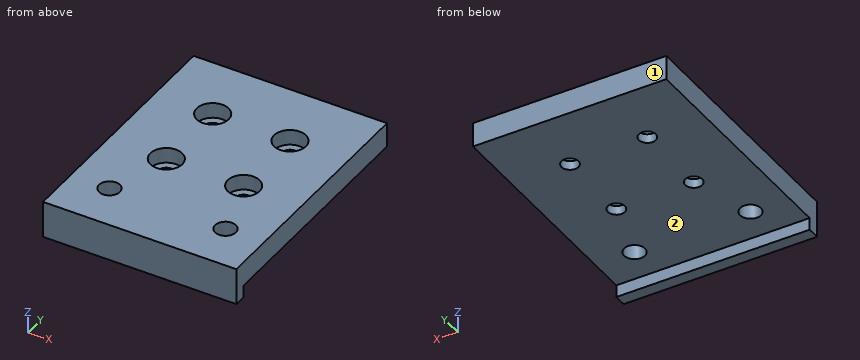
```python
from build123d import *

# Parameters (mm, degrees)
F0_W           = 50
F0_H           = 65
F1_DEPTH       = 9.525
F2_W           = 50
F2_H           = 61.825
F3_DEPTH       = 3.175
F5_D           = 4.4
F5_CBORE_D     = 8.25
F5_CBORE_DEPTH = 4
F7_D           = 5.4


# Not quite as in the source:
# - a length typed as a fraction of an inch, garbled in the dataset ("3 / 203.2 mm" for 3/8 in), is restored


with BuildPart() as f1:
    # F0 (on Top) → F1 (new body)
    with BuildSketch(Plane.XY):
        Rectangle(F0_W, F0_H)
    extrude(amount=F1_DEPTH)

    # F2 (on face) → F3 (cut)
    with BuildSketch(Plane(origin=(0, 0, 0), x_dir=(1, 0, 0), z_dir=(0, 0, -1))):
        with Locations((0, -1.5875)):
            Rectangle(F2_W, F2_H)
    extrude(amount=-F3_DEPTH, mode=Mode.SUBTRACT)

    # F5 (through all)
    with Locations(Plane.XY.offset(9.525)):
        with Locations((-10, 15.675), (10, 15.675), (10, -4.325), (-10, -4.325)):
            CounterBoreHole(F5_D / 2, F5_CBORE_D / 2, F5_CBORE_DEPTH)

    # F7 (through all)
    with Locations(Plane.XY.offset(9.525)):
        with Locations((-15, -20.5), (15, -20.5)):
            Hole(F7_D / 2)


solid = f1.part
```
Verification items for the finished model (mm, model axes). Face numbers are marked on the shaded views. A direction names the side the tool comes from. Coordinates: 2 decimals unless noted, no trailing zeros. Loops run counter-clockwise (first coordinate to the right, second up) from the corner with the lowest first, then second, coordinate; pieces in that order, holes last. Notation, with made-up numbers: (-24.75, -35.75) - (-11.75, -35.75) arc R22 cw to (-11.75, -29.75) - close; hole circle Ø7 at (-8.5, 29.25). An arc over 180 degrees is marked (long way). Answer as a JSON object with one key per item and string values.
(1) Access from +Z, -Z, +X, -X, +Y, -Y to the whole of each face (thin tool, end or side, straight path). Record for the marked faces 1 and 2.
Response:
{"face 1": "+Z, -Z, +X, -X, +Y", "face 2": "-Z, +X, -X, +Y"}
(2) Cross-section at D-D, the plane z = 4.5. Record the boundary of the cut face in (x, y) (3 decimals), then the cut area to 3 significant figures.
Response:
{"outline": "(-25, -32.5) - (25, -32.5) - (25, 32.5) - (-25, 32.5) - close; hole circle Ø5.4 at (-15, -20.5); hole circle Ø4.4 at (-10, -4.325); hole circle Ø4.4 at (-10, 15.675); hole circle Ø4.4 at (10, -4.325); hole circle Ø4.4 at (10, 15.675); hole circle Ø5.4 at (15, -20.5)", "area": "3,140 mm²"}
(3) Cross-section at A-A, the plane y = -20.5. Record the boundary of the cut face in (x, z) (3 decimals).
Response:
{"outline": "(-25, 3.175) - (-17.7, 3.175) - (-17.7, 9.525) - (-25, 9.525) - close; (-12.3, 3.175) - (12.3, 3.175) - (12.3, 9.525) - (-12.3, 9.525) - close; (17.7, 3.175) - (25, 3.175) - (25, 9.525) - (17.7, 9.525) - close"}
(4) Cross-section at B-B, the plane x = 10. Record the boundary of the cut face in (y, z) (3 decimals), then the cut area to 3 significant figures.
Response:
{"outline": "(-32.5, 0) - (-29.325, 0) - (-29.325, 3.175) - (-6.525, 3.175) - (-6.525, 5.525) - (-8.45, 5.525) - (-8.45, 9.525) - (-32.5, 9.525) - close; (-2.125, 3.175) - (13.475, 3.175) - (13.475, 5.525) - (11.55, 5.525) - (11.55, 9.525) - (-0.2, 9.525) - (-0.2, 5.525) - (-2.125, 5.525) - close; (17.875, 3.175) - (32.5, 3.175) - (32.5, 9.525) - (19.8, 9.525) - (19.8, 5.525) - (17.875, 5.525) - close", "area": "336 mm²"}
(5) Scan lines: line 1 along Y through (x, z) = (10, 7.4); line 2 along Y through (x, z) = (-15, 7.75); line 3 along X through (y, z) = (13, 6.5). Record each from-to range of solid material in increasing order.
Response:
{"line 1": "y = -32.5 to -8.45, -0.2 to 11.55, 19.8 to 32.5", "line 2": "y = -32.5 to -23.2, -17.8 to 32.5", "line 3": "x = -25 to -13.14, -6.86 to 6.86, 13.14 to 25"}
(6) Go/stop test with flat-tipped pins: pin 1 Ø6 at (x, y) = (-15, -20.5) entering from +Z (3 decimals); pin 2 Ø1 at (x, z) = (-3, 2.5) entering from +Y (3 decimals); pin 3 Ø2.5 at (x, y) = (10.5, -6) entering from +Z (3 decimals); pin 4 Ø12 at (x, y) = (-14, 13) entering from -Z (3 decimals). Record where each tip stops, or that it passes through.
Response:
{"pin 1": "stops at z = 9.525", "pin 2": "stops at y = -29.325", "pin 3": "stops at z = 5.525", "pin 4": "stops at z = 3.175"}
(7) Cross-section at C-C, the plane x = -15. Record the boundary of the cut face in (y, z) (3 decimals).
Response:
{"outline": "(-32.5, 0) - (-29.325, 0) - (-29.325, 3.175) - (-23.2, 3.175) - (-23.2, 9.525) - (-32.5, 9.525) - close; (-17.8, 3.175) - (32.5, 3.175) - (32.5, 9.525) - (-17.8, 9.525) - close"}
